The listing builds one solid part. Answer for the finished solid, in the listing's coordinates (mm). Face numbers are marked on the shaded views. A direction names the side the tool comes from. Give positions to 0.01 mm unless a question says otherwise; leave off trailing zeros. Write each loop counter-clockwise with the first axis right and the second up, starting at its lowest first coordinate (ties: lowest second). Pieces come first, ordered by that corner, then holes. Notation, with made-up numbers: (40, -36) - (60, -36) arc R26 cw to (60, -21) - close; hole circle Ø10 at (88.25, -4). An arc over 180 degrees is marked (long way). Return JSON: item names as keys, results as strings.
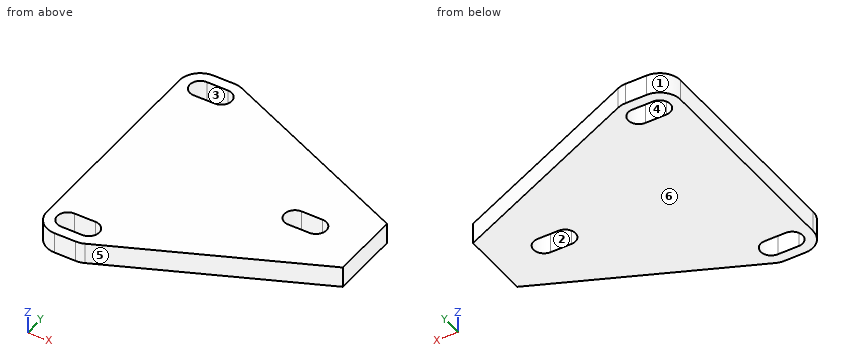
from build123d import *

# Parameters (mm, degrees)
BOSS_EXTRUDE1_DEPTH = 3


with BuildPart() as part:
    # Sketch1 → Boss-Extrude1 (new body)
    with BuildSketch(Plane.XY):
        with BuildLine():
            Line((31.5, -5), (31.5, 5))
            Line((31.5, 5), (2.714404574, 17.743213723))
            ThreePointArc((2.714404574, 17.743213723), (2.120628243, 17.935101461), (1.5, 18))
            Line((1.5, 18), (-1.5, 18))
            ThreePointArc((-1.5, 18), (-3.621320344, 17.121320344), (-4.5, 15))
            Line((-4.5, 15), (-4.5, -15))
            ThreePointArc((-4.5, -15), (-3.621320344, -17.121320344), (-1.5, -18))
            Line((-1.5, -18), (1.5, -18))
            ThreePointArc((1.5, -18), (2.120628243, -17.935101461), (2.714404574, -17.743213723))
            Line((2.714404574, -17.743213723), (31.5, -5))
        make_face()
        with BuildLine():
            Line((21.5, -1.5), (24.5, -1.5))
            ThreePointArc((24.5, -1.5), (26, 0), (24.5, 1.5))
            Line((24.5, 1.5), (21.5, 1.5))
            ThreePointArc((21.5, 1.5), (20, 0), (21.5, -1.5))
        make_face(mode=Mode.SUBTRACT)
        with BuildLine():
            Line((-1.5, 16.5), (1.5, 16.5))
            ThreePointArc((1.5, 16.5), (3, 15), (1.5, 13.5))
            Line((1.5, 13.5), (-1.5, 13.5))
            ThreePointArc((-1.5, 13.5), (-3, 15), (-1.5, 16.5))
        make_face(mode=Mode.SUBTRACT)
        with BuildLine():
            Line((1.5, -13.5), (-1.5, -13.5))
            ThreePointArc((-1.5, -13.5), (-3, -15), (-1.5, -16.5))
            Line((-1.5, -16.5), (1.5, -16.5))
            ThreePointArc((1.5, -16.5), (3, -15), (1.5, -13.5))
        make_face(mode=Mode.SUBTRACT)
    extrude(amount=BOSS_EXTRUDE1_DEPTH)


solid = part.part
Item 1: A cutting plane is placed at A-A on x = 1. Determine the outline of the cut face in (y, z), then the cut area to 3 significant figures.
Answer below:
{"outline": "(-18, 0) - (-16.5, 0) - (-16.5, 3) - (-18, 3) - close; (-13.5, 0) - (13.5, 0) - (13.5, 3) - (-13.5, 3) - close; (16.5, 0) - (18, 0) - (18, 3) - (16.5, 3) - close", "area": "90.0 mm²"}
Item 2: A cutting plane is placed at D-D on y = -10. Determine the outline of the cut face in (x, z), then the cut area to 3 significant figures.
Answer below:
{"outline": "(-4.5, 0) - (20.21, 0) - (20.21, 3) - (-4.5, 3) - close", "area": "74.1 mm²"}
Item 3: The mould has two halves that part along X. Classify the marked faces 3, 4, 5 and 6: +X half, -X half, draft (parallel to the pull), parting line (faces both ways), or undercut.
Answer below:
{"face 3": "undercut", "face 4": "undercut", "face 5": "+X half", "face 6": "draft"}
Item 4: For the marked faces 1 and 2, determine the directions among +Z, -Z, +X, -X, +Y, -Y from which every point of the face is accessible in a straight line to the end or side of a thin tool.
Answer below:
{"face 1": "+Z, -Z, -X, +Y", "face 2": "+Z, -Z"}
Item 5: Flat-ended cylindrical pins translate along their axes: P1, Ø1.5, axis at x = 23.5, z = 1.5, coming from the +Y side; P2, Ø0.9, axis at x = 23, z = 1.5, coming from the -Y side. Find the tip coordinate at first contact, or state that the pin passes through.
Answer below:
{"P1": "stops at y = 8.87", "P2": "stops at y = -8.96"}
Item 6: A cutting plane is placed at C-C on z = 2.25. Determine the outline of the cut face in (x, y).
Answer below:
{"outline": "(-4.5, -15) arc R3 ccw to (-1.5, -18) - (1.5, -18) arc R3 ccw to (2.71, -17.74) - (31.5, -5) - (31.5, 5) - (2.71, 17.74) arc R3 ccw to (1.5, 18) - (-1.5, 18) arc R3 ccw to (-4.5, 15) - close; hole (-1.5, -16.5) - (1.5, -16.5) arc R1.5 ccw to (1.5, -13.5) - (-1.5, -13.5) arc R1.5 ccw to start; hole (-1.5, 13.5) - (1.5, 13.5) arc R1.5 ccw to (1.5, 16.5) - (-1.5, 16.5) arc R1.5 ccw to start; hole (21.5, -1.5) - (24.5, -1.5) arc R1.5 ccw to (24.5, 1.5) - (21.5, 1.5) arc R1.5 ccw to start"}
Item 7: A cutting plane is placed at B-B on y = 0. Determine the outline of the cut face in (x, z).
Answer below:
{"outline": "(-4.5, 0) - (20, 0) - (20, 3) - (-4.5, 3) - close; (26, 0) - (31.5, 0) - (31.5, 3) - (26, 3) - close"}
Item 8: Consider L1, parallel to Y at x = -1, z = 0.45; L2, parallel to Y at x = 2.5, z = 2; L3, parallel to X at y = -1, z = 0.75. Determine where each line is inside the solid, lowest interval first.
Answer below:
{"L1": "y = -18 to -16.5, -13.5 to 13.5, 16.5 to 18", "L2": "y = -17.83 to -16.12, -13.88 to 13.88, 16.12 to 17.83", "L3": "x = -4.5 to 20.38, 25.62 to 31.5"}
